from build123d import *

# Parameters (mm, degrees)
F1_DEPTH = 40
F2_T     = -3
F3_W     = 110
F3_H     = 120
F4_DEPTH = 25


with BuildPart() as f1:
    # F0 (on Top) → F1 (new body)
    with BuildSketch(Plane.XY):
        with BuildLine():
            ThreePointArc((-69, -64), (-66.0710678119, -71.0710678119), (-59, -74))
            Line((-59, -74), (59, -74))
            ThreePointArc((59, -74), (66.0710678119, -71.0710678119), (69, -64))
            Line((69, -64), (69, 64))
            ThreePointArc((69, 64), (66.0710678119, 71.0710678119), (59, 74))
            Line((59, 74), (46.5, 74))
            Line((46.5, 74), (46.5, 144))
            ThreePointArc((46.5, 144), (43.5710678119, 151.0710678119), (36.5, 154))
            Line((36.5, 154), (-36.5, 154))
            ThreePointArc((-36.5, 154), (-43.5710678119, 151.0710678119), (-46.5, 144))
            Line((-46.5, 144), (-46.5, 74))
            Line((-46.5, 74), (-59, 74))
            ThreePointArc((-59, 74), (-66.0710678119, 71.0710678119), (-69, 64))
            Line((-69, 64), (-69, -64))
        make_face()
    extrude(amount=F1_DEPTH)

    # F2
    f2_openings = [f1.faces().sort_by_distance(p)[0] for p in [
        (0, 30.345732, 0),
    ]]
    offset(amount=F2_T, openings=f2_openings, kind=Kind.INTERSECTION)

    # F3 (on face) → F4 (cut)
    with BuildSketch(Plane(origin=(0, 0, 37), x_dir=(1, 0, 0), z_dir=(0, 0, -1))):
        Rectangle(F3_W, F3_H)
    extrude(amount=-F4_DEPTH, mode=Mode.SUBTRACT)


solid = f1.part
Geometry: final body of the model. Coordinates: model frame, mm. A direction names the side the tool comes from. Give positions to 0.01 mm unless a question says otherwise; leave off trailing zeros. Order: outer loops, then holes, each group sorted by start corner. A loop starts at its lowest first (then second) coordinate and runs counter-clockwise, first axis right, second up. Notation, with made-up numbers: (84.5, 77) -> (109.5, 77) arc R24 cw to (109.5, 111) -> close; hole circle Ø4 at (8.5, 63). An arc over 180 degrees is marked (long way). Answer as a JSON object with one key per item and string values.
Q1. Section A-A (x = 9.5). Output: boundary loops of the cut face in (y, z).
Entries:
{"outline": "(-74, 0) -> (-71, 0) -> (-71, 37) -> (-60, 37) -> (-60, 40) -> (-74, 40) -> close; (60, 37) -> (151, 37) -> (151, 0) -> (154, 0) -> (154, 40) -> (60, 40) -> close"}
Q2. Section B-B (y = 53.5). Output: boundary loops of the cut face in (x, z).
Entries:
{"outline": "(-69, 0) -> (-66, 0) -> (-66, 37) -> (-55, 37) -> (-55, 40) -> (-69, 40) -> close; (55, 37) -> (66, 37) -> (66, 0) -> (69, 0) -> (69, 40) -> (55, 40) -> close"}
Q3. Material intervals for probe 1 along X at (y, z) = (81, 6); probe 2 along X at (y, z) = (-21.5, 17); probe 3 along Y at (x, z) = (-14.5, 29), sorted ascending.
Entries:
{"probe 1": "x = -46.5 to -43.5, 43.5 to 46.5", "probe 2": "x = -69 to -66, 66 to 69", "probe 3": "y = -74 to -71, 151 to 154"}
Q4. First-contact query: pin 1 (11 mm diameter, centred on y = 115, z = 12.5, fed in from +X); pin 2 (18.5 mm diameter, centred on y = 110, z = 16, fed in from -X); pin 3 (10 mm diameter, centred on x = 52, z = 19, fed in from +Y). Flat tips, straight axial feed; report the tip coordinate or a pass-through.
Entries:
{"pin 1": "stops at x = 46.5", "pin 2": "stops at x = -46.5", "pin 3": "stops at y = 74"}
Q5. Section D-D (y = 106). Output: boundary loops of the cut face in (x, z).
Entries:
{"outline": "(-46.5, 0) -> (-43.5, 0) -> (-43.5, 37) -> (43.5, 37) -> (43.5, 0) -> (46.5, 0) -> (46.5, 40) -> (-46.5, 40) -> close"}
Q6. Section C-C (z = 15.5). Output: boundary loops of the cut face in (x, y).
Entries:
{"outline": "(-69, -64) arc R10 ccw to (-59, -74) -> (59, -74) arc R10 ccw to (69, -64) -> (69, 64) arc R10 ccw to (59, 74) -> (46.5, 74) -> (46.5, 144) arc R10 ccw to (36.5, 154) -> (-36.5, 154) arc R10 ccw to (-46.5, 144) -> (-46.5, 74) -> (-59, 74) arc R10 ccw to (-69, 64) -> close; hole (-66, -64) arc R7 ccw to (-59, -71) -> (59, -71) arc R7 ccw to (66, -64) -> (66, 64) arc R7 ccw to (59, 71) -> (43.5, 71) -> (43.5, 144) arc R7 ccw to (36.5, 151) -> (-36.5, 151) arc R7 ccw to (-43.5, 144) -> (-43.5, 71) -> (-59, 71) arc R7 ccw to (-66, 64) -> close"}
Q7. Draft query along X for faces 4 (the flat face through (-51, 71, 18)), 5 (the flat face through (46.5, 109, 20)), 6 (the cylindrical face through (64, 68.9, 18.2)), 7 (the flat face through (53, 74, 20)). Return one class per face: released by +X, released by -X, zero draft, split by the parting line, or undercut.
Entries:
{"face 4": "undercut", "face 5": "released by +X", "face 6": "undercut", "face 7": "zero draft"}
Q8. Access query for faces 1 (the cylindrical face through (-66.15, -70.99, 19.72)), 2 (the cylindrical face through (-41.4, 149, 18.2)), 3 (the flat face through (-53, 74, 20)). Directions: +Z, -Z, +X, -X, +Y, -Y. A direction counts if a zero-diameter tool reaches every point of the face in a straight line with its end or side. Return the directions, or none.
Entries:
{"face 1": "+Z, -Z, -X, -Y", "face 2": "-Z", "face 3": "+Z, -Z, -X, +Y"}
